from build123d import *

# Parameters (mm, degrees)
F0_W     = 132.152318
F0_H     = 72.699182
F0_W_2   = 122.152318
F0_H_2   = 62.699182
F1_DEPTH = 63.5
F2_R     = 8.194556
F3_DEPTH = 132.153319
F4_W     = 58.48376
F4_H     = 20.056372
F5_DEPTH = 72.700182


with BuildPart() as f1:
    # F0 (on Top) → F1 (new body)
    with BuildSketch(Plane.XY):
        Rectangle(F0_W, F0_H)
        Rectangle(F0_W_2, F0_H_2, mode=Mode.SUBTRACT)
    extrude(amount=F1_DEPTH)

    # F2 (on face) → F3 (cut, through all)
    with BuildSketch(Plane.YZ.offset(66.076159)):
        with Locations((0, 31.75)):
            Circle(F2_R)
    extrude(amount=-F3_DEPTH, mode=Mode.SUBTRACT)

    # F4 (on face) → F5 (cut, through all)
    with BuildSketch(Plane.XZ.offset(36.349591)):
        with Locations((0, 53.471814)):
            Rectangle(F4_W, F4_H)
    extrude(amount=-F5_DEPTH, mode=Mode.SUBTRACT)


solid = f1.part
The listing builds one solid part. Answer for the finished solid, in the listing's coordinates (mm). A direction names the side the tool comes from. Round coordinates to 2 decimals unless told otherwise and drop trailing zeros. Order: outer loops, then holes, each group sorted by start corner. A loop starts at its lowest first (then second) coordinate and runs counter-clockwise, first axis right, second up. Notation, with made-up numbers: (5, 27) -> (28, 27) arc R12 cw to (28, 37) -> close; hole circle Ø5 at (-38, -19). An arc over 180 degrees is marked (long way). One line per item, written item: value.
Item 1: Find section A-A, the plane z = 31.75. Give the vertices of the cut face in (x, y).
Taken from the geometry:
outline: (-66.08, -36.35) -> (66.08, -36.35) -> (66.08, -8.19) -> (61.08, -8.19) -> (61.08, -31.35) -> (-61.08, -31.35) -> (-61.08, -8.19) -> (-66.08, -8.19) -> close; (-66.08, 8.19) -> (-61.08, 8.19) -> (-61.08, 31.35) -> (61.08, 31.35) -> (61.08, 8.19) -> (66.08, 8.19) -> (66.08, 36.35) -> (-66.08, 36.35) -> close
Item 2: For a pull along X with two mould halves and no side action, classify faces 4 (the flat face through (63, -3, 63.5)), 5 (the flat face through (66.076, -9, 31)), 6 (the flat face through (0, -34, 43.444)) as released by +X, released by -X, zero draft, split by the parting line, or undercut.
Taken from the geometry:
face 4: zero draft
face 5: released by +X
face 6: undercut
Item 3: For faces 1 (the cylindrical face through (-63.541, 4.405, 38.66)), 2 (the flat face through (-29.242, -34, 53)), 3 (the flat face through (-1, 31.35, 24)), determine the directions among +Z, -Z, +X, -X, +Y, -Y from which every point of the face is accessible in a straight line to the end or side of a thin tool.
Taken from the geometry:
face 1: +X, -X
face 2: +Z, +Y, -Y
face 3: +Z, -Z
Item 4: Find section C-C, the plane y = 0. Give the vertices of the cut face in (x, z).
Taken from the geometry:
outline: (-66.08, 0) -> (-61.08, 0) -> (-61.08, 23.56) -> (-66.08, 23.56) -> close; (-66.08, 39.94) -> (-61.08, 39.94) -> (-61.08, 63.5) -> (-66.08, 63.5) -> close; (61.08, 0) -> (66.08, 0) -> (66.08, 23.56) -> (61.08, 23.56) -> close; (61.08, 39.94) -> (66.08, 39.94) -> (66.08, 63.5) -> (61.08, 63.5) -> close
Item 5: Straight lines are drawn through the part: L1, parallel to X at y = -27.5, z = 32; L2, parallel to Y at x = -37.5, z = 34.5; L3, parallel to Z at x = 63, y = 0. For each, find the intervals that lie inside material, in ascending order.
Taken from the geometry:
L1: x = -66.08 to -61.08, 61.08 to 66.08
L2: y = -36.35 to -31.35, 31.35 to 36.35
L3: z = 0 to 23.56, 39.94 to 63.5
Item 6: Given P1, Ø2.5, axis at x = 3.5, y = -35, coming from the +Z side, flat-ended and moving along its own axis, determine where the tip first touches the part or whether it passes through.
Taken from the geometry:
P1: stops at z = 43.44
Item 7: Find section D-D, the plane z = 11. Give the vertices of the cut face in (x, y), then the cut area to 3 significant figures.
Taken from the geometry:
outline: (-66.08, -36.35) -> (66.08, -36.35) -> (66.08, 36.35) -> (-66.08, 36.35) -> close; hole (-61.08, -31.35) -> (61.08, -31.35) -> (61.08, 31.35) -> (-61.08, 31.35) -> close
area: 1,950 mm2
Item 8: Find section B-B, the plane x = 51.5. Give the vertices of the cut face in (y, z), then the cut area to 3 significant figures.
Taken from the geometry:
outline: (-36.35, 0) -> (-31.35, 0) -> (-31.35, 63.5) -> (-36.35, 63.5) -> close; (31.35, 0) -> (36.35, 0) -> (36.35, 63.5) -> (31.35, 63.5) -> close
area: 635 mm2
